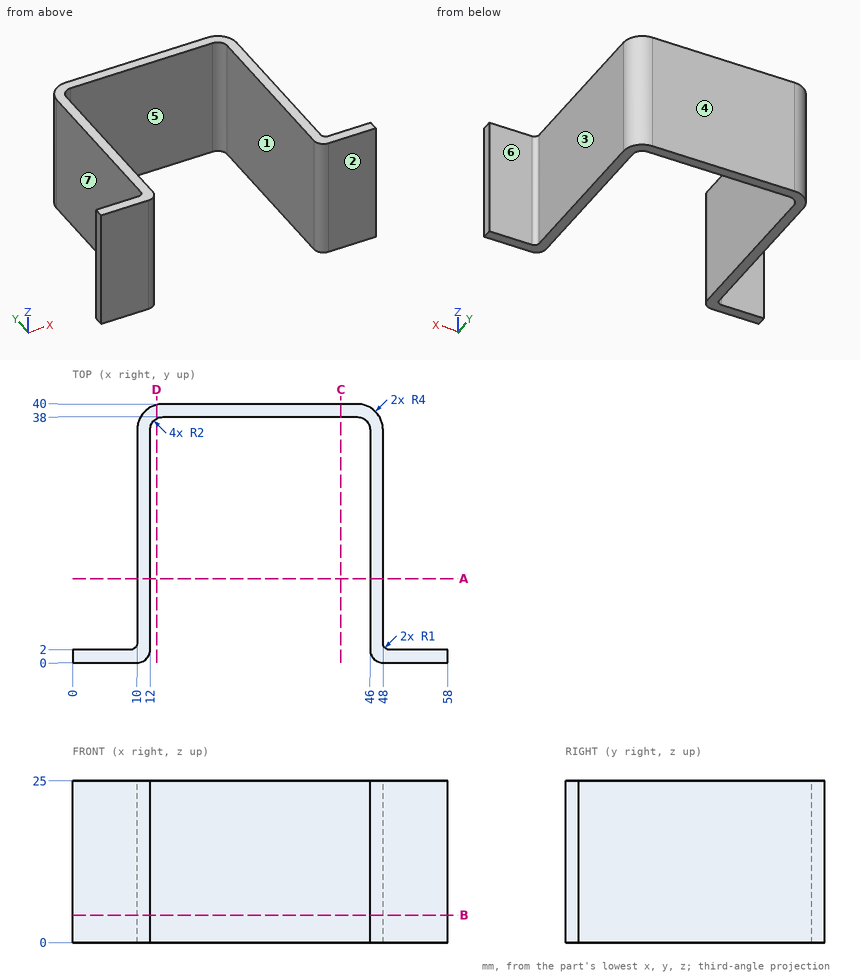
Study the drawing (mm; zero at the part's minimum x, y, z) and answer. A direction names the side the tool comes from. Coordinates: 2 decimals unless noted, no trailing zeros. Write each loop counter-clockwise with the first axis right and the second up, starting at its lowest first coordinate (ties: lowest second). Pieces come first, ordered by that corner, then holes. Notation, with made-up numbers: (-33.5, 14) - (-2.5, 14) arc R25 ccw to (-2.5, 35) - close; hole circle Ø1 at (-7.5, -13). An arc over 180 degrees is marked (long way). Return JSON: item names as keys, results as strings. Group by question number.
1. A cutting plane is placed at D-D, the plane x = 13. Determine the outline of the cut face in (y, z), plus the area to 3 significant figures.
2. A cutting plane is placed at B-B, the plane z = 4.25. Determine the outline of the cut face in (x, y).
3. Straight lines are drawn through the part: L1, parallel to X at y = 24, z = 20.25; L2, parallel to Y at x = 49, z = 21.25; L3, parallel to Y at x = 39, z = 1.75. For each, find the intervals that lie inside material, in ascending order.
4. Which of the six approach directions +Z, -Z, +X, -X, +Y, -Y give full straight-line access (tool end or side, diameter ignored) to the marked faces 4, 5, 6 and 7?
5. A cutting plane is placed at A-A, the plane y = 13. Determine the outline of the cut face in (x, z), plus the area to 3 significant figures.
6. A cutting plane is placed at C-C, the plane x = 41.5. Determine the outline of the cut face in (y, z).
7. Determine the mould class of the marked faces 1, 2 and 3 for opening direction X: released by +X, released by -X, zero draft, split by the parting line, or undercut.
8. Given pin 1 (10 mm diameter, centred on x = 4.5, z = 18.5, fed in from +Y); pin 2 (4.5 mm diameter, centred on x = 55.5, z = 10.5, fed in from +Y); pin 3 (12 mm diameter, centred on y = 9, z = 4.5, fed in from +X), each flat-ended and moving along its own axis, determine where each tip first touches the part or whether it passes through.
Ans:
{
 "1": {"outline": "(37.73, 0) - (39.87, 0) - (39.87, 25) - (37.73, 25) - close", "area": "53.5 mm²"},
 "2": {"outline": "(0, 0) - (10, 0) arc R2 ccw to (12, 2) - (12, 36) arc R2 cw to (14, 38) - (44, 38) arc R2 cw to (46, 36) - (46, 2) arc R2 ccw to (48, 0) - (58, 0) - (58, 2) - (49, 2) arc R1 cw to (48, 3) - (48, 36) arc R4 ccw to (44, 40) - (14, 40) arc R4 ccw to (10, 36) - (10, 3) arc R1 cw to (9, 2) - (0, 2) - close"},
 "3": {"L1": "10 to 12, 46 to 48", "L2": "0 to 2", "L3": "38 to 40"},
 "4": {"face 4": "+Z, -Z, +X, -X, +Y", "face 5": "+Z, -Z, -Y", "face 6": "+Z, -Z, +X, +Y", "face 7": "+Z, -Z, -X, +Y"},
 "5": {"outline": "(10, 0) - (12, 0) - (12, 25) - (10, 25) - close; (46, 0) - (48, 0) - (48, 25) - (46, 25) - close", "area": "100 mm²"},
 "6": {"outline": "(38, 0) - (40, 0) - (40, 25) - (38, 25) - close"},
 "7": {"face 1": "undercut", "face 2": "zero draft", "face 3": "released by +X"},
 "8": {"pin 1": "y = 2.13", "pin 2": "y = 2", "pin 3": "x = 48"}
}
